```python
from build123d import *

# Parameters (mm, degrees)
F0_W     = 76.2685239315
F0_H     = 25.6147123873
F1_DEPTH = 76.2
F3_W     = 153.1126648188
F3_H     = 50.6538152695
F4_DEPTH = 76.2
F5_W     = 77.4197503924
F5_H     = 25.9025208652
F6_DEPTH = 76.2


with BuildPart() as f1:
    # F0 (on Front) → F1 (new body)
    with BuildSketch(Plane.XZ):
        with Locations((38.1342619658, 12.8073561937)):
            Rectangle(F0_W, F0_H)
    extrude(amount=F1_DEPTH)


with BuildPart() as f4:
    # F3 (on Front) → F4 (new body)
    with BuildSketch(Plane.XZ):
        with Locations((0.8634179831, 25.3269076347)):
            Rectangle(F3_W, F3_H)
    extrude(amount=-F4_DEPTH)

    # F5 (on face) → F6 (cut, through all)
    with BuildSketch(Plane.XZ):
        with Locations((38.7098751962, 37.7025548369)):
            Rectangle(F5_W, F5_H)
    extrude(amount=-F6_DEPTH, mode=Mode.SUBTRACT)


solid = f4.part
```
Can you work these out from the model? Positions are in its coordinate system, mm. A direction names the side the tool comes from. Coordinates: 2 decimals unless noted, no trailing zeros. Order: outer loops, then holes, each group sorted by start corner. A loop starts at its lowest first (then second) coordinate and runs counter-clockwise, first axis right, second up.
1. If we section it at B-B (z = 30.5): Please give me the cut outline in (x, y).
2. If we section it at A-A (y = 27): Please give me the cut outline in (x, z), then the cut area to 3 significant figures.
3. For faces 1 (the face through (77.42, 38, 12)), 2 (the face through (0, 38, 38)), which set-ups out of +Z, -Z, +X, -X, +Y, -Y let a thin tool reach every point of the face, with its end or its side?
4. I need wall thicknesses on line 1 (X direction, y = 55, z = 36); line 2 (Z direction, x = 2, y = 20.5). Which ranges of each line are inside material? Lowest first, please.
5. If we section it at C-C (x = 44): Please give me the cut outline in (y, z), then the cut area to 3 significant figures.
Entries:
1. outline: (-75.69, 0) - (0, 0) - (0, 76.2) - (-75.69, 76.2) - close
2. outline: (-75.69, 0) - (77.42, 0) - (77.42, 24.75) - (0, 24.75) - (0, 50.65) - (-75.69, 50.65) - close
2. area: 5,750 mm2
3. face 1: +Z, -Z, +X, +Y, -Y
3. face 2: +Z, +X, +Y, -Y
4. line 1: x = -75.69 to 0
4. line 2: z = 0 to 24.75
5. outline: (0, 0) - (76.2, 0) - (76.2, 24.75) - (0, 24.75) - close
5. area: 1,890 mm2
